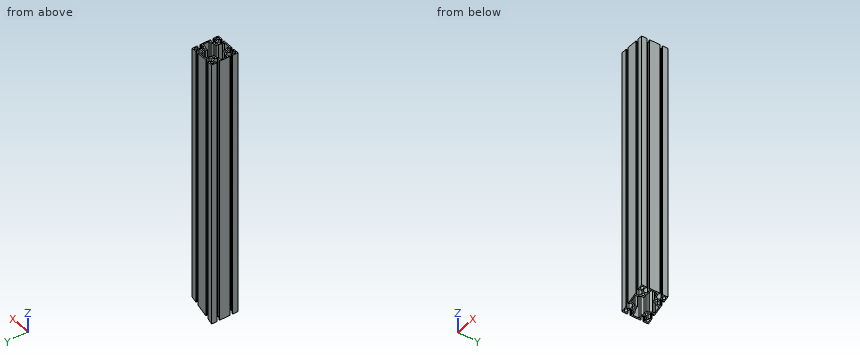
```python
from build123d import *

# Parameters (mm, degrees)
F0_R          = 3
F0_R_2        = 2.5
F1_DEPTH      = 618.33
F2_R          = 2
F3_R          = 7
F5_DEPTH      = 30
F5_DEPTH_BACK = 30


# Not quite as in the source:
# - a feature names something its author has since deleted; it is built from what else it names


with BuildPart() as f1:
    # F0 (on Top) → F1 (new body)
    with BuildSketch(Plane.XY):
        with BuildLine():
            Line((18.15, -30), (30, -30))
            Line((30, -30), (30, -18.15))
            Line((30, -18.15), (27.5, -18.15))
            Line((27.5, -18.15), (27.5, -20.15))
            Line((27.5, -20.15), (21.5477069044, -20.15))
            ThreePointArc((21.5477069044, -20.15), (19.5, -15), (21.5477069044, -9.85))
            Line((21.5477069044, -9.85), (27.5, -9.85))
            Line((27.5, -9.85), (27.5, -11.85))
            Line((27.5, -11.85), (30, -11.85))
            Line((30, -11.85), (30, 11.85))
            Line((30, 11.85), (27.5, 11.85))
            Line((27.5, 11.85), (27.5, 9.85))
            Line((27.5, 9.85), (21.5477069044, 9.85))
            ThreePointArc((21.5477069044, 9.85), (19.5, 15), (21.5477069044, 20.15))
            Line((21.5477069044, 20.15), (27.5, 20.15))
            Line((27.5, 20.15), (27.5, 18.15))
            Line((27.5, 18.15), (30, 18.15))
            Line((30, 18.15), (30, 30))
            Line((30, 30), (18.15, 30))
            Line((18.15, 30), (18.15, 27.5))
            Line((18.15, 27.5), (20.15, 27.5))
            Line((20.15, 27.5), (20.15, 21.5477069044))
            ThreePointArc((20.15, 21.5477069044), (15, 19.5), (9.85, 21.5477069044))
            Line((9.85, 21.5477069044), (9.85, 27.5))
            Line((9.85, 27.5), (11.85, 27.5))
            Line((11.85, 27.5), (11.85, 30))
            Line((11.85, 30), (-11.85, 30))
            Line((-11.85, 30), (-11.85, 27.5))
            Line((-11.85, 27.5), (-9.85, 27.5))
            Line((-9.85, 27.5), (-9.85, 21.5477069044))
            ThreePointArc((-9.85, 21.5477069044), (-15, 19.5), (-20.15, 21.5477069044))
            Line((-20.15, 21.5477069044), (-20.15, 27.5))
            Line((-20.15, 27.5), (-18.15, 27.5))
            Line((-18.15, 27.5), (-18.15, 30))
            Line((-18.15, 30), (-30, 30))
            Line((-30, 30), (-30, 18.15))
            Line((-30, 18.15), (-27.5, 18.15))
            Line((-27.5, 18.15), (-27.5, 20.15))
            Line((-27.5, 20.15), (-21.5477069044, 20.15))
            ThreePointArc((-21.5477069044, 20.15), (-19.5, 15), (-21.5477069044, 9.85))
            Line((-21.5477069044, 9.85), (-27.5, 9.85))
            Line((-27.5, 9.85), (-27.5, 11.85))
            Line((-27.5, 11.85), (-30, 11.85))
            Line((-30, 11.85), (-30, -11.85))
            Line((-30, -11.85), (-27.5, -11.85))
            Line((-27.5, -11.85), (-27.5, -9.85))
            Line((-27.5, -9.85), (-21.5477069044, -9.85))
            ThreePointArc((-21.5477069044, -9.85), (-19.5, -15), (-21.5477069044, -20.15))
            Line((-21.5477069044, -20.15), (-27.5, -20.15))
            Line((-27.5, -20.15), (-27.5, -18.15))
            Line((-27.5, -18.15), (-30, -18.15))
            Line((-30, -18.15), (-30, -30))
            Line((-30, -30), (-18.15, -30))
            Line((-18.15, -30), (-18.15, -27.5))
            Line((-18.15, -27.5), (-20.15, -27.5))
            Line((-20.15, -27.5), (-20.15, -21.5477069044))
            ThreePointArc((-20.15, -21.5477069044), (-15, -19.5), (-9.85, -21.5477069044))
            Line((-9.85, -21.5477069044), (-9.85, -27.5))
            Line((-9.85, -27.5), (-11.85, -27.5))
            Line((-11.85, -27.5), (-11.85, -30))
            Line((-11.85, -30), (11.85, -30))
            Line((11.85, -30), (11.85, -27.5))
            Line((11.85, -27.5), (9.85, -27.5))
            Line((9.85, -27.5), (9.85, -21.5477069044))
            ThreePointArc((9.85, -21.5477069044), (15, -19.5), (20.15, -21.5477069044))
            Line((20.15, -21.5477069044), (20.15, -27.5))
            Line((20.15, -27.5), (18.15, -27.5))
            Line((18.15, -27.5), (18.15, -30))
        make_face()
        with Locations((-25, -25)):
            Circle(F0_R, mode=Mode.SUBTRACT)
        with Locations((-15, -15)):
            Circle(F0_R_2, mode=Mode.SUBTRACT)
        with Locations((25, -25)):
            Circle(F0_R, mode=Mode.SUBTRACT)
        with Locations((15, -15)):
            Circle(F0_R_2, mode=Mode.SUBTRACT)
        with Locations((-25, 25)):
            Circle(F0_R, mode=Mode.SUBTRACT)
        with Locations((-15, 15)):
            Circle(F0_R_2, mode=Mode.SUBTRACT)
        Polygon((-7, 22), (-7, 27.5), (0, 27.5), (7, 27.5), (7, 22), (10, 16), (10, 10), (16, 10), (22, 7), (27.5, 7), (27.5, 0), (27.5, -7), (22, -7), (16, -10), (10, -10), (10, -16), (7, -22), (7, -27.5), (0, -27.5), (-7, -27.5), (-7, -22), (-10, -16), (-10, -10), (-16, -10), (-22, -7), (-27.5, -7), (-27.5, 0), (-27.5, 7), (-22, 7), (-16, 10), (-10, 10), (-10, 16), align=None, mode=Mode.SUBTRACT)
        with Locations((15, 15)):
            Circle(F0_R_2, mode=Mode.SUBTRACT)
        with Locations((25, 25)):
            Circle(F0_R, mode=Mode.SUBTRACT)
    extrude(amount=F1_DEPTH)

    # F2
    f2_edges = [f1.edges().sort_by_distance(p)[0] for p in [
        (-7, 27.5, 309.165),
        (7, 27.5, 309.165),
    ]]
    fillet(f2_edges, radius=F2_R)

    # F3
    f3_edges = [f1.edges().sort_by_distance(p)[0] for p in [
        (-10, 16, 309.165),
        (10, 16, 309.165),
    ]]
    fillet(f3_edges, radius=F3_R)

    # F4 (on Front) → F5 (cut, two sides)
    with BuildSketch(Plane.XZ) as f5_sk:
        Polygon((227.6837248597, 106.7360936397), (-30, 0), (35.1751396755, -157.3467061341), (292.8588645352, -50.6106124944), align=None)
    extrude(amount=F5_DEPTH, mode=Mode.SUBTRACT)
    extrude(f5_sk.sketch, amount=-F5_DEPTH_BACK, mode=Mode.SUBTRACT)


solid = f1.part
```
Build history of the part. All positions in model axes, mm. Round coordinates to 2 decimals unless told otherwise and drop trailing zeros. Order: outer loops, then holes, each group sorted by start corner. A loop starts at its lowest first (then second) coordinate and runs counter-clockwise, first axis right, second up. Notation, with made-up numbers: (55, -11.75) -> (65, -11.75) arc R13 ccw to (65, 10.25) -> close; hole circle Ø9 at (-16.75, -13). An arc over 180 degrees is marked (long way). Answer in a Markdown table with one row per item.
1) Band-saw the part on B-B on z = 279.5. Give the number of separate pieces and of enclosed holes in the cut face, and give its area (3 significant figures).
Values:
| item | result |
|---|---|
| separate pieces | 1 |
| enclosed holes | 9 |
| area | 1,080 mm2 |
2) Pin check, flat tips, straight feed: P1, Ø4, axis at x = -9, y = 19.5, coming from the -Z side; P2, Ø9.5, axis at x = 25, y = -25, coming from the -Z side; P3, Ø5, axis at y = 13, z = 402, coming from the +X side; P4, Ø1, axis at x = -16, z = 158.5, coming from the +Y side. Stop position of each tip, or through.
Values:
| item | result |
|---|---|
| P1 | z = 7.87 |
| P2 | z = 20.81 |
| P3 | x = 30 |
| P4 | y = 19.65 |
3) Wall check: L1, parallel to X at y = -25, z = 458; L2, parallel to X at y = 15, z = 355.5. Give the ranges that are in metal, low to high.
Values:
| item | result |
|---|---|
| L1 | -30 to -28, -22 to -20.15, -9.85 to -7, 7 to 9.85, 20.15 to 22, 28 to 30 |
| L2 | -19.5 to -17.5, -12.5 to -9.97, 9.97 to 12.5, 17.5 to 19.5 |
4) Band-saw the part on A-A on x = 0. Give the cut face in (y, z), and give its area (3 significant figures).
Values:
| item | result |
|---|---|
| outline | (-30, 12.43) -> (-27.5, 12.43) -> (-27.5, 618.33) -> (-30, 618.33) -> close; (27.5, 12.43) -> (30, 12.43) -> (30, 618.33) -> (27.5, 618.33) -> close |
| area | 3,030 mm2 |
